Autodesk Inventor part; units mm, degrees
ref_plane "YZ Plane" through (0, 0, 0) normal (1, 0, 0) x (0, 1, 0)
ref_plane "XZ Plane" through (0, 0, 0) normal (0, 1, 0) x (-1, 0, 0)
ref_plane "XY Plane" through (0, 0, 0) normal (0, 0, 1) x (1, 0, 0)
sketch "Sketch1" plane through (0, 0, 0) normal (0, 1, 0) x (-1, 0, 0)
  line L0 (15.875, 20.1549) -> (-15.875, 20.1549) construction
  line L1 (14.478, 18.7579) -> (-14.478, 18.7579) construction
  line L2 (-14.478, 21.5519) -> (14.478, 21.5519) construction
  arc A0 (14.478, 18.7579) -> (14.478, 21.5519) centre (14.478, 20.1549) ccw construction
  arc A1 (-14.478, 21.5519) -> (-14.478, 18.7579) centre (-14.478, 20.1549) ccw construction
  line L3 (25.4, -25.4) -> (-25.4, -25.4)
  line L4 (-25.4, -25.4) -> (-25.4, 25.4)
  line L5 (-25.4, 25.4) -> (25.4, 25.4)
  line L6 (25.4, 25.4) -> (25.4, -25.4)
  line L7 (25.4, -25.4) -> (-25.4, 25.4) construction
  line L8 (-25.4, -25.4) -> (25.4, 25.4) construction
  line L9 (-15.875, -20.1549) -> (15.875, -20.1549) construction
  line L10 (-14.478, -18.7579) -> (14.478, -18.7579) construction
  line L11 (14.478, -21.5519) -> (-14.478, -21.5519) construction
  arc A2 (-14.478, -18.7579) -> (-14.478, -21.5519) centre (-14.478, -20.1549) ccw construction
  arc A3 (14.478, -21.5519) -> (14.478, -18.7579) centre (14.478, -20.1549) ccw construction
  line L12 (0, -20.1549) -> (0, 20.1549) construction
  line L13 (-17.3355, -4.699) -> (-17.3355, 4.699) construction
  line L14 (-15.875, -3.2385) -> (-15.875, 3.2385) construction
  line L15 (-18.796, 3.2385) -> (-18.796, -3.2385) construction
  arc A4 (-18.796, -3.2385) -> (-15.875, -3.2385) centre (-17.3355, -3.2385) ccw construction
  arc A5 (-15.875, 3.2385) -> (-18.796, 3.2385) centre (-17.3355, 3.2385) ccw construction
  line L16 (-14.478, -21.2979) -> (14.478, -21.2979)
  arc A6 (14.478, -21.2979) -> (14.478, -19.0119) centre (14.478, -20.1549) ccw
  line L17 (14.478, -19.0119) -> (-14.478, -19.0119)
  arc A7 (-14.478, -19.0119) -> (-14.478, -21.2979) centre (-14.478, -20.1549) ccw
  line L18 (-14.478, 19.0119) -> (14.478, 19.0119)
  arc A8 (14.478, 19.0119) -> (14.478, 21.2979) centre (14.478, 20.1549) ccw
  line L19 (14.478, 21.2979) -> (-14.478, 21.2979)
  arc A9 (-14.478, 21.2979) -> (-14.478, 19.0119) centre (-14.478, 20.1549) ccw
  line L20 (-16.129, 3.2385) -> (-16.129, -3.2385)
  arc A10 (-18.542, -3.2385) -> (-16.129, -3.2385) centre (-17.3355, -3.2385) ccw
  line L21 (-18.542, -3.2385) -> (-18.542, 3.2385)
  arc A11 (-16.129, 3.2385) -> (-18.542, 3.2385) centre (-17.3355, 3.2385) ccw
  point P0 (0, 0)
  point P1 (0, 0)
  point P2 (-17.3355, 0)
  point P3 (-15.875, -20.1549)
  dimension "d0" = 31.75
  dimension "d1" = 50.8
  dimension "d2" = 50.8
  dimension "d3" = 37.5158
  dimension "d4" = 2.794
  dimension "d5" = 31.75
  dimension "d6" = 2.794
  dimension "d7" = 9.398
  dimension "d8" = 2.921
  dimension "clear" = 0.254
  dimension "d10" = 0.254
  dimension "d11" = 0.254
extrude "Extrusion1" add sketch "Sketch1" along normal blind 3.175 contours L3 L4 L5 L6 | A7 L17 A6 L16 | A9 L19 A8 L18 | L20 A10 L21 A11
extrude "Extrusion2" add sketch "Sketch1" against normal blind 38.1 contours A7 L17 A6 L16 | A9 L19 A8 L18 | L20 A10 L21 A11
fillet "Fillet1" radius 3.175 4 edges at (25.4, 1.5875, 25.4) (-25.4, 1.5875, 25.4) (25.4, 1.5875, -25.4) (-25.4, 1.5875, -25.4)
fillet "Fillet2" radius 3.175 12 edges at (0, 0, -21.2979) (-15.621, 0, -20.1549) (0, 0, -19.0119) (15.621, 0, -20.1549) (17.3355, 0, 4.445) (18.542, 0, 0) (17.3355, 0, -4.445) (16.129, 0, 0) (-15.621, 0, 20.1549) (0, 0, 21.2979) (15.621, 0, 20.1549) (0, 0, 19.0119)
equation "\"d5\" = d0"
equation "\"d6\" = d4"
equation "\"d10\" = clear"
equation "\"d11\" = clear"
properties part number "vrm tool" material "ABS Plastic"
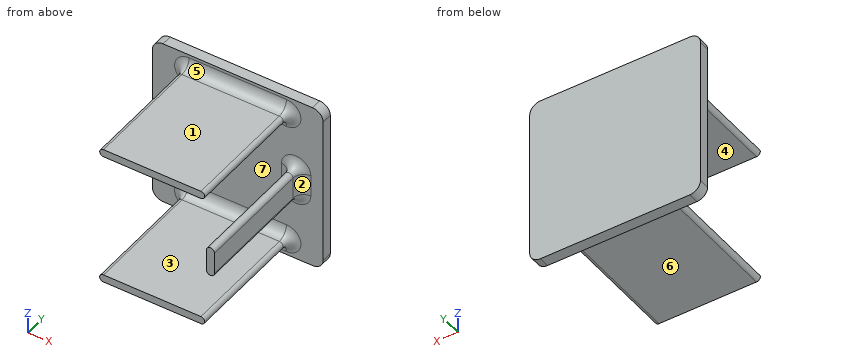
The listing builds one solid part. Answer for the finished solid, in the listing's coordinates (mm). Face numbers are marked on the shaded views. A direction names the side the tool comes from. Round coordinates to 2 decimals unless told otherwise and drop trailing zeros. Write each loop counter-clockwise with the first axis right and the second up, starting at its lowest first coordinate (ties: lowest second). Pieces come first, ordered by that corner, then holes. Notation, with made-up numbers: M 24,47 L 73,47 A25 cw 73,61 Z; hole C -3,45.25 d3. An arc over 180 degrees is marked long. Write each question's results on one line, items separated by ' | '. Start each with the question number.
Item 1: Which of the six approach directions +Z, -Z, +X, -X, +Y, -Y give full straight-line access (tool end or side, diameter ignored) to the marked faces 1, 2 and 3?
Item 2: Find section C-C on x = 2. Write down the section's boundary in (y, z) (3 decimals).
Item 3: The mould has two halves that part along Z. Classify the marked faces 4, 5, 6 and 7: +Z half, -Z half, draft (parallel to the pull), parting line (faces both ways), or undercut.
Item 4: Given pin 1 Ø8 at (x, y) = (-9, -10.5) entering from +Z; pin 2 Ø3 at (y, z) = (-15.5, 0) entering from -X; pin 3 Ø12 at (x, y) = (4.5, -15.5) entering from -Z; pin 4 Ø2 at (y, z) = (-19, -5.5) entering from +X, each flat-ended and moving along its own axis, determine where each tip first touches the part or whether it passes through.
Item 5: Find section B-B on z = -2. Write down the section's boundary in (x, y) (3 decimals).
Item 6: Straight lines are drawn through the part: probe 1 along Z at (x, y) = (-6.5, -13); probe 2 along Z at (x, y) = (17.5, -5); probe 3 along Y at (x, z) = (-3, -11) (3 decimals). For each, find the intervals that lie inside material, in ascending order.
Item 7: Find section A-A on y = -31. Write down the section's boundary in (x, z), and give its area (3 significant figures).
Item 8: Find section D-D on y = -1. Write down the section's boundary in (x, z) (1 decimal).
Answer block:
1) face 1: +Z, +X, -X, -Y | face 2: +Z, -Z, +X, -Y | face 3: +X, -X, -Y
2) outline: M -38.1,-21.298 L -3.175,-21.298 A3.175 cw 0,-24.473 L 0,-25.4 L 3.175,-25.4 L 3.175,25.4 L 0,25.4 L 0,24.473 A3.175 cw -3.175,21.298 L -38.1,21.298 L -38.1,19.012 L -3.175,19.012 A3.175 cw 0,15.837 L 0,-15.837 A3.175 cw -3.175,-19.012 L -38.1,-19.012 Z
3) face 4: undercut | face 5: +Z half | face 6: -Z half | face 7: undercut
4) pin 1: stops at z = 21.3 | pin 2: stops at x = 16.13 | pin 3: stops at z = -21.3 | pin 4: passes through
5) outline: M -25.4,0 L 12.954,0 A3.175 cw 16.129,-3.175 L 16.129,-38.1 L 18.542,-38.1 L 18.542,-3.175 A3.175 cw 21.717,0 L 25.4,0 L 25.4,3.175 L -25.4,3.175 Z
6) probe 1: z = -21.3 to -19.01, 19.01 to 21.3 | probe 2: z = -4.43 to 4.43 | probe 3: y = 0 to 3.175
7) outline: M -14.48,-21.3 L 14.48,-21.3 A1.14 ccw 14.48,-19.01 L -14.48,-19.01 A1.14 ccw Z; M -14.48,19.01 L 14.48,19.01 A1.14 ccw 14.48,21.3 L -14.48,21.3 A1.14 ccw Z; M 16.13,-3.24 A1.21 ccw 18.54,-3.24 L 18.54,3.24 A1.21 ccw 16.13,3.24 Z | area: 161 mm²
8) outline: M -14.5,-22.2 L 14.5,-22.2 A2 ccw 14.5,-18.1 L -14.5,-18.1 A2 ccw Z; M -14.5,18.1 L 14.5,18.1 A2 ccw 14.5,22.2 L -14.5,22.2 A2 ccw Z; M 15.3,-3.2 A2.1 ccw 19.4,-3.2 L 19.4,3.2 A2.1 ccw 15.3,3.2 Z
